```python
from build123d import *

# Parameters (mm, degrees)
F0_R     = 1
F1_DEPTH = 1.56
F2_DEPTH = 1.2
F3_DEPTH = 0.82
F4_DEPTH = 0.4
F5_R     = 0.3


with BuildPart() as f1:
    # F0 (on Top) → F1 (new body)
    with BuildSketch(Plane.XY):
        Circle(F0_R)
    extrude(amount=F1_DEPTH)

    # F0 (on Top) → F2 (join)
    with BuildSketch(Plane.XY):
        Polygon((0.85, 1.85), (-0.85, 1.85), (-1.85, 0.85), (-1.85, -0.85), (-0.85, -1.85), (0.85, -1.85), (1.85, -0.85), (1.85, 0.85), align=None)
        Circle(F0_R, mode=Mode.SUBTRACT)
    extrude(amount=F2_DEPTH)

    # F0 (on Top) → F3 (join)
    with BuildSketch(Plane.XY):
        Polygon((1.25, 2.5), (-1.25, 2.5), (-1.65, 2.1), (-2.15, 1.6), (-2.5, 1.25), (-2.5, -1.25), (-2.15, -1.6), (-1.65, -2.1), (-1.25, -2.5), (1.25, -2.5), (1.65, -2.1), (2.15, -1.6), (2.5, -1.25), (2.5, 1.25), (2.15, 1.6), (1.65, 2.1), align=None)
        Polygon((-1.85, 0.85), (-0.85, 1.85), (0.85, 1.85), (1.85, 0.85), (1.85, -0.85), (0.85, -1.85), (-0.85, -1.85), (-1.85, -0.85), align=None, mode=Mode.SUBTRACT)
    extrude(amount=F3_DEPTH)

    # F0 (on Top) → F4 (join)
    with BuildSketch(Plane.XY):
        Polygon((-2.15, 1.6), (-1.65, 2.1), (-3.2, 2.1), (-3.2, 1.6), align=None)
        Polygon((-1.65, -2.1), (-2.15, -1.6), (-3.2, -1.6), (-3.2, -2.1), align=None)
        Polygon((3.2, -1.6), (2.15, -1.6), (1.65, -2.1), (3.2, -2.1), align=None)
        Polygon((3.2, 2.1), (1.65, 2.1), (2.15, 1.6), (3.2, 1.6), align=None)
    extrude(amount=F4_DEPTH)

    # F5
    f5_edges = [f1.edges().sort_by_distance(p)[0] for p in [
        (-1.35, 1.35, 1.2),
        (-1.85, 0, 1.2),
        (-1.35, -1.35, 1.2),
        (0, -1.85, 1.2),
        (1.35, -1.35, 1.2),
        (1.85, 0, 1.2),
        (1.35, 1.35, 1.2),
        (0, 1.85, 1.2),
        (-1.875, 1.875, 0.82),
        (-2.5, 0, 0.82),
        (-1.875, -1.875, 0.82),
        (0, -2.5, 0.82),
        (1.875, -1.875, 0.82),
        (2.5, 0, 0.82),
        (1.875, 1.875, 0.82),
        (0, 2.5, 0.82),
        (-3.2, 1.85, 0.4),
        (-3.2, -1.85, 0.4),
        (3.2, -1.85, 0.4),
        (3.2, 1.85, 0.4),
    ]]
    fillet(f5_edges, radius=F5_R)


solid = f1.part
```
Geometry: final body of the model. Coordinates: model frame, mm. A direction names the side the tool comes from. Give positions to 0.01 mm unless a question says otherwise; leave off trailing zeros. Loops run counter-clockwise (first coordinate to the right, second up) from the corner with the lowest first, then second, coordinate; pieces in that order, holes last. Notation, with made-up numbers: (13.25, -29.75) -> (21.25, -29.75) arc R17 ccw to (21.25, -0.75) -> close; hole circle Ø6 at (32, -25.75). An arc over 180 degrees is marked (long way). Return JSON: item names as keys, results as strings.
Item 1: Line query: line 1 (X direction, y = -0.35, z = 0.3); line 2 (Z direction, x = 1.25, y = 1.5); line 3 (Z direction, x = -1.25, y = 1). Output: solid intervals per line, ascending.
Filled in:
{"line 1": "-2.5 to 2.5", "line 2": "0 to 0.82", "line 3": "0 to 1.2"}
Item 2: Access query for faces 1 (the flat face through (-1, 1, 1.2)), 2 (the cylindrical face through (1.3, -1.28, 1.11)). Directions: +Z, -Z, +X, -X, +Y, -Y. A direction counts if a zero-diameter tool reaches every point of the face in a straight line with its end or side. Return the directions, or none.
Filled in:
{"face 1": "+Z", "face 2": "+Z, +X, -Y"}
Item 3: Section B-B, the plane y = 0.6. Output: boundary loops of the cut face in (x, z), plus the area to 3 significant figures.
Filled in:
{"outline": "(-2.5, 0) -> (2.5, 0) -> (2.5, 0.52) arc R0.3 ccw to (2.2, 0.82) -> (1.85, 0.82) -> (1.85, 0.9) arc R0.3 ccw to (1.55, 1.2) -> (0.8, 1.2) -> (0.8, 1.56) -> (-0.8, 1.56) -> (-0.8, 1.2) -> (-1.55, 1.2) arc R0.3 ccw to (-1.85, 0.9) -> (-1.85, 0.82) -> (-2.2, 0.82) arc R0.3 ccw to (-2.5, 0.52) -> close", "area": "6.00 mm^2"}
Item 4: Section A-A, the plane x = 0. Output: boundary loops of the cut face in (y, z).
Filled in:
{"outline": "(-2.5, 0) -> (2.5, 0) -> (2.5, 0.52) arc R0.3 ccw to (2.2, 0.82) -> (1.85, 0.82) -> (1.85, 0.9) arc R0.3 ccw to (1.55, 1.2) -> (1, 1.2) -> (1, 1.56) -> (-1, 1.56) -> (-1, 1.2) -> (-1.55, 1.2) arc R0.3 ccw to (-1.85, 0.9) -> (-1.85, 0.82) -> (-2.2, 0.82) arc R0.3 ccw to (-2.5, 0.52) -> close"}
Item 5: Section C-C, the plane z = 1.35. Output: boundary loops of the cut face in (x, y).
Filled in:
{"outline": "circle Ø2 at (0, 0)"}
